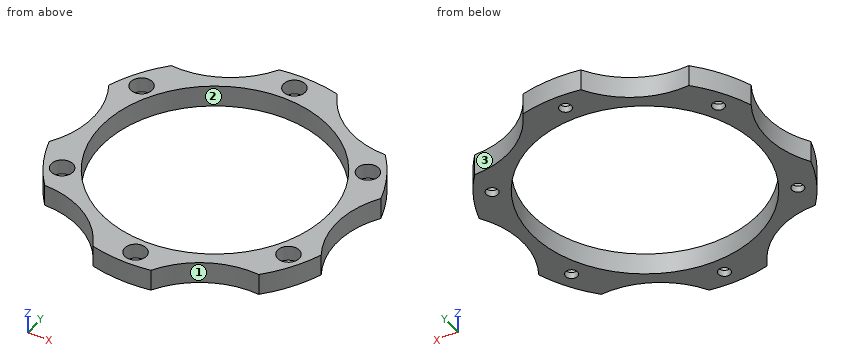
from build123d import *

# Parameters (mm, degrees)
IZIM1_R                     = 67.5
IZIM1_R_2                   = 52.5
IZIM1_R_3                   = 2.75
Y_KSEKLIK_EKSTR_ZYON1_DEPTH = 10
KES_EKSTR_ZYON1_DEPTH       = 14
IZIM3_R                     = 5
KES_EKSTR_ZYON2_DEPTH       = 7


with BuildPart() as part:
    # Çizim1 → Yükseklik-Ekstrüzyon1 (new body)
    with BuildSketch(Plane.XY):
        Circle(IZIM1_R)
        Circle(IZIM1_R_2, mode=Mode.SUBTRACT)
        with Locations((0, 60)):
            Circle(IZIM1_R_3, mode=Mode.SUBTRACT)
        with Locations((51.961524227, 30)):
            Circle(IZIM1_R_3, mode=Mode.SUBTRACT)
        with Locations((51.961524227, -30)):
            Circle(IZIM1_R_3, mode=Mode.SUBTRACT)
        with Locations((0, -60)):
            Circle(IZIM1_R_3, mode=Mode.SUBTRACT)
        with Locations((-51.961524227, -30)):
            Circle(IZIM1_R_3, mode=Mode.SUBTRACT)
        with Locations((-51.961524227, 30)):
            Circle(IZIM1_R_3, mode=Mode.SUBTRACT)
    extrude(amount=Y_KSEKLIK_EKSTR_ZYON1_DEPTH)

    # Çizim2 → Kes-Ekstrüzyon1 (cut)
    with BuildSketch(Plane(origin=(0, 0, 0), x_dir=(-1, 0, 0), z_dir=(0, 0, -1))):
        with BuildLine():
            Line((-61.212117231, 43.852600407), (-15, 68.50053352))
            ThreePointArc((-15, 68.50053352), (-33.51113221, 47.561593986), (-61.212117231, 43.852600407))
        make_face()
        with BuildLine():
            Line((7.371407359, 74.937548745), (51.823202201, 47.240647817))
            ThreePointArc((51.823202201, 47.240647817), (24.433982531, 52.802288797), (7.371407359, 74.937548745))
        make_face()
        with BuildLine():
            Line((68.58352459, 31.084948338), (66.823202201, -21.259885703))
            ThreePointArc((66.823202201, -21.259885703), (57.945114741, 5.240694811), (68.58352459, 31.084948338))
        make_face()
        with BuildLine():
            Line((61.212117231, -43.852600407), (15, -68.50053352))
            ThreePointArc((15, -68.50053352), (33.51113221, -47.561593986), (61.212117231, -43.852600407))
        make_face()
        with BuildLine():
            Line((-7.371407359, -74.937548745), (-51.823202201, -47.240647817))
            ThreePointArc((-51.823202201, -47.240647817), (-24.433982531, -52.802288797), (-7.371407359, -74.937548745))
        make_face()
        with BuildLine():
            Line((-68.58352459, -31.084948338), (-66.823202201, 21.259885703))
            ThreePointArc((-66.823202201, 21.259885703), (-57.945114741, -5.240694811), (-68.58352459, -31.084948338))
        make_face()
    extrude(amount=-KES_EKSTR_ZYON1_DEPTH, mode=Mode.SUBTRACT)

    # Çizim3 → Kes-Ekstrüzyon2 (cut)
    with BuildSketch(Plane.XY.offset(10)):
        with Locations((0, 60)):
            Circle(IZIM3_R)
        with Locations((51.961524227, 30)):
            Circle(IZIM3_R)
        with Locations((51.961524227, -30)):
            Circle(IZIM3_R)
        with Locations((0, -60)):
            Circle(IZIM3_R)
        with Locations((-51.961524227, -30)):
            Circle(IZIM3_R)
        with Locations((-51.961524227, 30)):
            Circle(IZIM3_R)
    extrude(amount=-KES_EKSTR_ZYON2_DEPTH, mode=Mode.SUBTRACT)


solid = part.part
The model under review builds one solid part; all positions refer to its coordinate system, in mm. Face numbers are marked on the shaded views. Give positions to 0.01 mm unless a question says otherwise; leave off trailing zeros. Loops run counter-clockwise (first coordinate to the right, second up) from the corner with the lowest first, then second, coordinate; pieces in that order, holes last. Notation, with made-up numbers: (47.25, 89) -> (96.25, 89) arc R27 ccw to (96.25, 112) -> close; hole circle Ø11 at (23.25, -7.5). An arc over 180 degrees is marked (long way). Put each result on its own line as item: value. Start each with the question number.
1. We need section A-A on x = 0. State the section outline as (y, z) points, then the cut area to 3 significant figures.
2. We need section D-D on y = -30. State the section outline as (x, z) points.
3. Wall thickness on probe 1 along Y at (x, z) = (0, 5.5); probe 2 along X at (y, z) = (-34.5, 4); probe 3 along Y at (x, z) = (48, 3.25): over which ranges is each line inside the solid? List them lowest first.
4. We need section C-C on y = 3.5. State the section outline as (x, z) points, then the cut area to 3 significant figures.
5. Clearance check with flat-ended pins moving along their axes: P1, Ø11.5, axis at x = 0, y = -60, coming from the -Z side; P2, Ø4, axis at x = 14.5, z = 2.5, coming from the +Y side; P3, Ø4, axis at y = -38, z = 9, coming from the -X side; P4, Ø6, axis at x = 0, y = 60, coming from the +Z side. State where each tip first meets the part, or that it passes through.
6. Mouldability with a two-part tool opening along Y and no side actions: class the marked faces 1, 2 and 3 as released by +Y, released by -Y, zero draft, split by the parting line, or undercut.
7. We need section B-B on z = 8. State the section outline as (x, y) points (3 decimals).
Determined:
1. outline: (-67.5, 0) -> (-62.75, 0) -> (-62.75, 3) -> (-65, 3) -> (-65, 10) -> (-67.5, 10) -> close; (-57.25, 0) -> (-52.5, 0) -> (-52.5, 10) -> (-55, 10) -> (-55, 3) -> (-57.25, 3) -> close; (52.5, 0) -> (57.25, 0) -> (57.25, 3) -> (55, 3) -> (55, 10) -> (52.5, 10) -> close; (62.75, 0) -> (67.5, 0) -> (67.5, 10) -> (65, 10) -> (65, 3) -> (62.75, 3) -> close
1. area: 127 mm^2
2. outline: (-60.47, 0) -> (-54.71, 0) -> (-54.71, 3) -> (-56.96, 3) -> (-56.96, 10) -> (-60.47, 10) -> close; (-49.21, 0) -> (-43.08, 0) -> (-43.08, 10) -> (-46.96, 10) -> (-46.96, 3) -> (-49.21, 3) -> close; (43.08, 0) -> (49.21, 0) -> (49.21, 3) -> (46.96, 3) -> (46.96, 10) -> (43.08, 10) -> close; (54.71, 0) -> (60.47, 0) -> (60.47, 10) -> (56.96, 10) -> (56.96, 3) -> (54.71, 3) -> close
3. probe 1: -67.5 to -65, -55 to -52.5, 52.5 to 55, 65 to 67.5
3. probe 2: -58.02 to -54.14, -49.78 to -39.57, 39.57 to 49.78, 54.14 to 58.02
3. probe 3: -46.82 to -33.05, -26.95 to -21.27, 21.27 to 26.95, 33.05 to 43.09
4. outline: (-57.92, 0) -> (-52.38, 0) -> (-52.38, 10) -> (-57.92, 10) -> close; (52.38, 0) -> (58.61, 0) -> (58.61, 10) -> (52.38, 10) -> close
4. area: 118 mm^2
5. P1: z = 0
5. P2: y = 66.33
5. P3: x = -57.1
5. P4: z = 3
6. face 1: released by -Y
6. face 2: undercut
6. face 3: released by +Y
7. outline: (-64.875, -18.64) arc R67.5 ccw to (-52.15, -42.856) arc R40 cw to (-16.295, -65.504) arc R67.5 ccw to (11.039, -66.591) arc R40 cw to (48.58, -46.864) arc R67.5 ccw to (63.189, -23.736) arc R40 cw to (64.875, 18.64) arc R67.5 ccw to (52.15, 42.856) arc R40 cw to (16.295, 65.504) arc R67.5 ccw to (-11.039, 66.591) arc R40 cw to (-48.58, 46.864) arc R67.5 ccw to (-63.189, 23.736) arc R40 cw to start; hole circle Ø10 at (-51.962, -30); hole circle Ø10 at (-51.962, 30); hole circle Ø105 at (0, 0); hole circle Ø10 at (0, -60); hole circle Ø10 at (0, 60); hole circle Ø10 at (51.962, -30); hole circle Ø10 at (51.962, 30)
